Here's the drawing with two shaded views (mm, measured from the low corner). I have some questions. A direction names the side the tool comes from. Give positions to 0.01 mm unless a question says otherwise; leave off trailing zeros. Loops run counter-clockwise (first coordinate to the right, second up) from the corner with the lowest first, then second, coordinate; pieces in that order, holes last. Notation, with made-up numbers: (-24.5, 2.25) -> (6.5, 2.25) arc R31 cw to (6.5, 32.25) -> close; hole circle Ø6 at (19, 61.25). An arc over 180 degrees is marked (long way). Answer in a Markdown table with one row per item. Add a question column.
Item 1: If we section it at C-C (x = 34): Write out the boundary of the cut face in (y, z).
Item 2: If we section it at A-A (z = 24.5): Write out the boundary of the cut face in (x, y), then the cut area to 3 significant figures.
Item 3: If I drill on line 1 (Y direction, x = 275, z = 68); line 2 (X direction, y = 161, z = 42); line 3 (Z direction, x = 136.5, y = 133.5), over which ranges is the centre line in solid material (lowest first)?
Item 4: Which directions (+Z, -Z, +X, -X, +Y, -Y) give clear straight access to the entire face, cutting with the end or side of a thin tool? Please do the marked faces 1 and 2.
Item 5: For P1, Ø8, axis at y = 104.5, z = 69, coming from the -X side; P2, Ø8, axis at x = 138.5, y = 90.5, coming from the -Z side, each with a flat end and sliding along its axis, tell me the tip position at first contact or that it passes through.
Item 6: If we section it at B-B (y = 138.5): Write out the boundary of the cut face in (x, z), then the cut area to 3 significant figures.
Item 7: We'd pull the mould along Y, two halves only. Please class the marked faces 3, 4 and 5: released by +Y, released by -Y, zero draft, split by the parting line, or undercut.
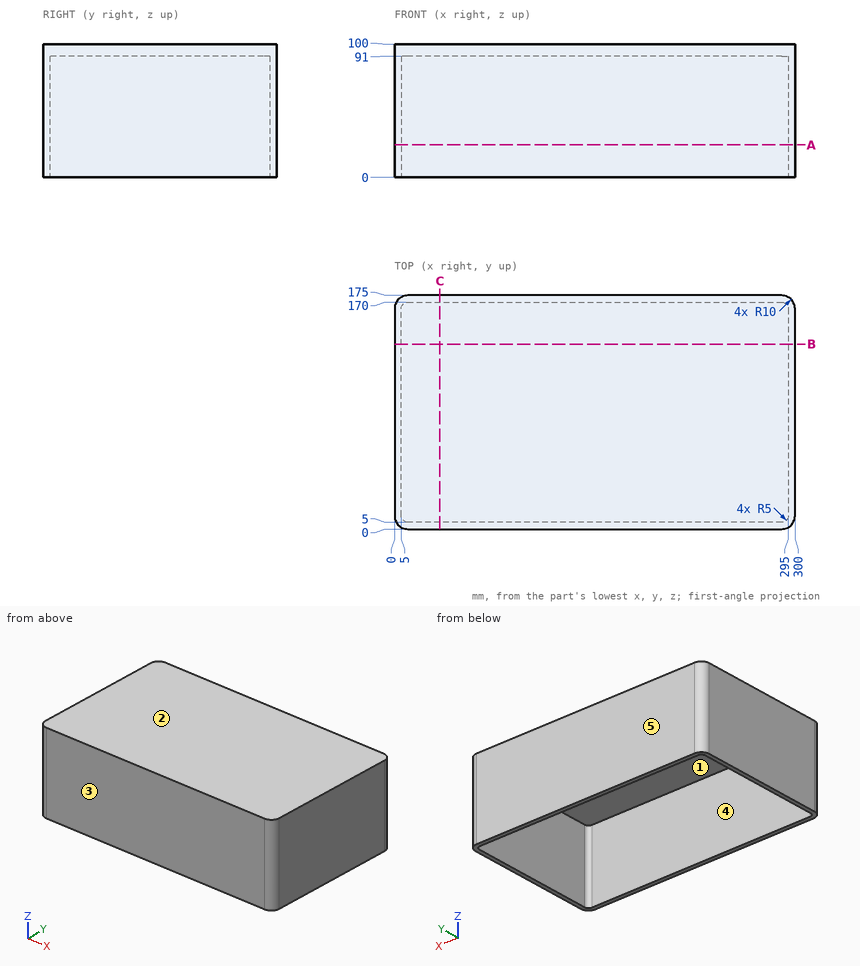
Recorded:
| question | item | result |
|---|---|---|
| 1 | outline | (0, 0) -> (5, 0) -> (5, 91) -> (170, 91) -> (170, 0) -> (175, 0) -> (175, 100) -> (0, 100) -> close |
| 2 | outline | (0, 10) arc R10 ccw to (10, 0) -> (290, 0) arc R10 ccw to (300, 10) -> (300, 165) arc R10 ccw to (290, 175) -> (10, 175) arc R10 ccw to (0, 165) -> close; hole (5, 10) arc R5 ccw to (10, 5) -> (290, 5) arc R5 ccw to (295, 10) -> (295, 165) arc R5 ccw to (290, 170) -> (10, 170) arc R5 ccw to (5, 165) -> close |
| 2 | area | 4,590 mm^2 |
| 3 | line 1 | y = 0 to 5, 170 to 175 |
| 3 | line 2 | x = 0 to 5, 295 to 300 |
| 3 | line 3 | z = 91 to 100 |
| 4 | face 1 | -Z |
| 4 | face 2 | +Z, +X, -X, +Y, -Y |
| 5 | P1 | stops at x = 0 |
| 5 | P2 | stops at z = 91 |
| 6 | outline | (0, 0) -> (5, 0) -> (5, 91) -> (295, 91) -> (295, 0) -> (300, 0) -> (300, 100) -> (0, 100) -> close |
| 6 | area | 3,610 mm^2 |
| 7 | face 3 | released by -Y |
| 7 | face 4 | undercut |
| 7 | face 5 | released by +Y |
